Source: CAD feature listing. Evaluate the final solid. Frame: model axes, mm. Face numbers are marked on the shaded views. A direction names the side the tool comes from. Round coordinates to 2 decimals unless told otherwise and drop trailing zeros. Order: outer loops, then holes, each group sorted by start corner. A loop starts at its lowest first (then second) coordinate and runs counter-clockwise, first axis right, second up. Notation, with made-up numbers: M 68.5,79.5 L 110.5,79.5 A19 cw 110.5,102.5 Z; hole C 50.5,68.5 d1. An arc over 180 degrees is marked long. Answer as CSV lines item,"result". Start each with the question number.
Item 1: Section query B-B on x = -56. Return the cut outline in (y, z).
Item 2: Line query: line 1 (X direction, y = 10, z = 43.5); line 2 (Z direction, x = -39, y = 27); line 3 (Y direction, x = -25.5, z = 11). Output: solid intervals per line, ascending. Write a range as [from, to].
Item 3: Section query C-C on y = -8. Return the cut outline in (x, z), plus the area to 3 significant figures.
Item 4: Section query A-A on z = 7.5. Return the cut outline in (x, y), plus the area to 3 significant figures.
Item 5: First-contact query: P1, Ø23, axis at x = -26, z = 17, coming from the +Y side; P2, Ø23, axis at x = -32, y = 16.5, coming from the +Z side; P3, Ø14, axis at y = 20.5, z = 25.5, coming from the +X side; P4, Ø1, axis at x = -23, y = -9.5, coming from the +Z side. Flat tips, straight axial feed; report the tip coordinate or a pass-through.
Item 6: Pull-direction query (X, two-part tool) for the marked faces 4, 5, 6 and 7; classes: +X half, -X half, draft (parallel to the pull), parting line (faces both ways), or undercut.
Item 7: Set-up query: the marked faces 1, 2 and 3. Return all of +Z, -Z, +X, -X, +Y, -Y with unobstructed straight access to the full face (end or side cutting, diameter ignored); none if empty.
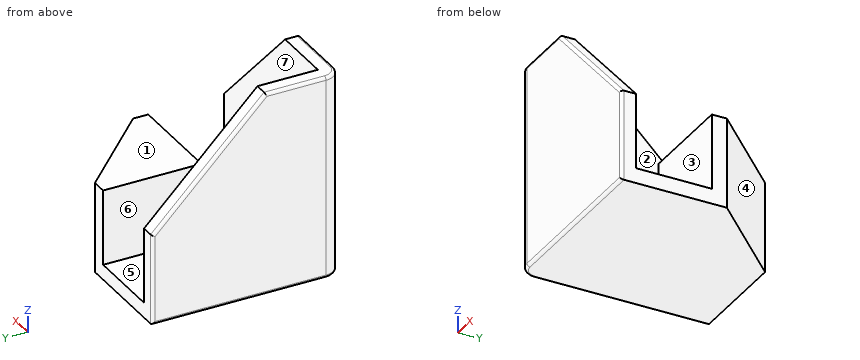
from build123d import *

# Parameters (mm, degrees)
F1_DEPTH     = 24
F3_DEPTH     = 20
F4_DEPTH     = 30
F6_DEPTH     = 25
F8_DEPTH     = 25
F9_R         = 0.8
F10_T1_DEPTH = 54
F10_T4_ANGLE = 90
F10_T6_ANGLE = 90


# Not quite as in the source:
# - a fillet or chamfer that OpenCascade refuses, or shapes differently, is made with other operations: its cross-section is extruded or revolved along the edge and cut away or added


with BuildPart() as f1:
    # F0 (on Top) → F1 (new body)
    with BuildSketch(Plane.XY):
        Polygon((-36.005956176, 35.1195232451), (-64.005956176, 35.1195232451), (-64.005956176, -14.8804767549), (-14.005956176, -14.8804767549), (-14.005956176, 13.1195232451), align=None)
    extrude(amount=F1_DEPTH)

    # F2 (on face) → F3 (cut)
    with BuildSketch(Plane.XY.offset(24)):
        Polygon((-40.005956176, 35.1195232451), (-60.005956176, 35.1195232451), (-60.005956176, -10.8804767549), (-14.005956176, -10.8804767549), (-14.005956176, 9.1195232451), (-40.005956176, 9.1195232451), align=None)
    extrude(amount=-F3_DEPTH, mode=Mode.SUBTRACT)

    # F4 (add): a face of the model
    f4_faces = [f1.faces().sort_by_distance(p)[0] for p in [
        (-60.7130629571, 12.1195232451, 24),
    ]]
    extrude(f4_faces, amount=F4_DEPTH)

    # F5 (on face) → F6 (cut)
    with BuildSketch(Plane.XZ.offset(14.8804767549)):
        Polygon((-14.005956176, 24), (-14.005956176, 54), (-44.005956176, 54), align=None)
    extrude(amount=-F6_DEPTH, mode=Mode.SUBTRACT)

    # F7 (on face) → F8 (cut)
    with BuildSketch(Plane(origin=(-64.005956176, 0, 0), x_dir=(0, -1, 0), z_dir=(-1, 0, 0))):
        Polygon((-5.1195232451, 54), (-35.1195232451, 54), (-35.1195232451, 24), align=None)
    extrude(amount=-F8_DEPTH, mode=Mode.SUBTRACT)

    # F9
    f9_edges = [f1.edges().sort_by_distance(p)[0] for p in [
        (-64.005956, -4.880477, 54),
        (-54.005956, -14.880477, 54),
        (-64.005956, 20.119523, 39),
        (-29.005956, -14.880477, 39),
        (-64.005956, 35.119523, 12),
        (-14.005956, -14.880477, 12),
        (-64.005956, 10.119523, 0),
        (-39.005956, -14.880477, 0),
    ]]
    fillet(f9_edges, radius=F9_R)

    # F10: fillet of radius 4 on 1 edges, made by hand

    # F10_s2 → F10_t1 (cut)
    with BuildSketch(Plane.XY):
        with BuildLine():
            ThreePointArc((-64.005956176, -10.8804767549), (-62.8343833007, -13.7089038797), (-60.005956176, -14.8804767549))
            Line((-60.005956176, -14.8804767549), (-64.005956176, -14.8804767549))
            Line((-64.005956176, -14.8804767549), (-64.005956176, -10.8804767549))
        make_face()
    extrude(amount=F10_T1_DEPTH, mode=Mode.SUBTRACT)

    # F10_s3 → F10_t4 (revolve, cut)
    with BuildSketch(Plane.YZ.offset(-60.005956176)):
        with BuildLine():
            ThreePointArc((-14.0804767549, 0), (-14.6461621799, 0.2343145751), (-14.8804767549, 0.8))
            Line((-14.8804767549, 0.8), (-14.8804767549, 0))
            Line((-14.8804767549, 0), (-14.0804767549, 0))
        make_face()
    revolve(axis=Axis((-60.005956176, -10.8804767549, 0), (0, 0, -1)), revolution_arc=F10_T4_ANGLE, mode=Mode.SUBTRACT)

    # F10_s5 → F10_t6 (revolve, cut)
    with BuildSketch(Plane.XZ.offset(10.8804767549)):
        with BuildLine():
            ThreePointArc((-63.205956176, 54), (-63.7716416009, 53.7656854249), (-64.005956176, 53.2))
            Line((-64.005956176, 53.2), (-64.005956176, 54))
            Line((-64.005956176, 54), (-63.205956176, 54))
        make_face()
    revolve(axis=Axis((-60.005956176, -10.8804767549, 54), (0, 0, 1)), revolution_arc=F10_T6_ANGLE, mode=Mode.SUBTRACT)


solid = f1.part
Results:
1,outline,"M -14.88,0.8 A0.8 ccw -14.08,0 L 35.12,0 L 35.12,4 L -10.88,4 L -10.88,54 L -14.08,54 A0.8 ccw -14.88,53.2 Z"
2,line 1,"[-64.01, -60.01]"
2,line 2,"[0, 24]"
2,line 3,"[-14.88, -10.88], [9.12, 24.61]"
3,outline,"M -64.01,0.8 A0.8 ccw -63.21,0 L -14.01,0 L -14.01,4 L -60.01,4 L -60.01,54 L -63.21,54 A0.8 ccw -64.01,53.2 Z"
3,area,"400 mm^2"
4,outline,"M -64.01,-10.88 A4 ccw -60.01,-14.88 L -14.81,-14.88 A0.8 ccw -14.01,-14.08 L -14.01,-10.88 L -60.01,-10.88 L -60.01,35.12 L -63.21,35.12 A0.8 ccw -64.01,34.32 Z; M -40.01,9.12 L -14.01,9.12 L -14.01,13.12 L -36.01,35.12 L -40.01,35.12 Z"
4,area,"814 mm^2"
5,P1,"y = 35.12"
5,P2,"z = 24"
5,P3,"x = -14.55"
5,P4,"z = 4"
6,face 4,"+X half"
6,face 5,"undercut"
6,face 6,"undercut"
6,face 7,"draft"
7,face 1,"+Z, +X, +Y"
7,face 2,"+Z, +Y"
7,face 3,"+Z, +X"
